from build123d import *

# Parameters (mm, degrees)
SKETCH1_R           = 11.2
SKETCH1_R_2         = 13
SKETCH1_R_3         = 1.45
SKETCH1_R_4         = 2.2
BOSS_EXTRUDE1_DEPTH = 5
BOSS_EXTRUDE2_DEPTH = 33
SKETCH1_4_R         = 13
SKETCH1_4_R_2       = 9.6
SKETCH1_4_R_3       = 8.6
SKETCH1_4_R_4       = 6
BOSS_EXTRUDE3_DEPTH = 3
SKETCH1_5_R         = 13
SKETCH1_5_R_2       = 9.6
SKETCH1_5_R_3       = 8.6
BOSS_EXTRUDE4_DEPTH = 8
SKETCH1_6_R         = 13
SKETCH1_6_R_2       = 9.6
BOSS_EXTRUDE5_DEPTH = 10
SKETCH2_R           = 2.2
CUT_EXTRUDE1_DEPTH  = 10
CHAMFER1_SIZE       = 4
CHAMFER2_SIZE       = 5


with BuildPart() as part:
    # Sketch1 → Boss-Extrude1 (new body)
    # profile 1 of 2: a face of its own
    with BuildSketch(Plane(origin=(0, 0, 0), x_dir=(1, 0, 0), z_dir=(0, 1, 0))):
        Polygon((-45, -45), (-45, -24), (-45, -21.4), (-71.4, -21.4), (-71.4, 21.4), (-45, 21.4), (-45, 24), (-45, 45), (45, 45), (45, 21), (76, 21), (76, -21), (45, -21), (45, -45), align=None)
        with Locations(Location((55, 0, 0), (0, 0, 270))):
            Circle(SKETCH1_R, mode=Mode.SUBTRACT)
        with Locations(Location((0, 0, 0), (0, 0, 270))):
            Circle(SKETCH1_R_2, mode=Mode.SUBTRACT)
        with Locations(Location((39.5, -15.5, 0), (0, 0, 270))):
            Circle(SKETCH1_R_3, mode=Mode.SUBTRACT)
        with Locations(Location((-35, -35, 0), (0, 0, 270))):
            Circle(SKETCH1_R_4, mode=Mode.SUBTRACT)
        with Locations(Location((-35, 35, 0), (0, 0, 270))):
            Circle(SKETCH1_R_4, mode=Mode.SUBTRACT)
        with Locations(Location((35, 35, 0), (0, 0, 270))):
            Circle(SKETCH1_R_4, mode=Mode.SUBTRACT)
        with Locations(Location((39.5, 15.5, 0), (0, 0, 270))):
            Circle(SKETCH1_R_3, mode=Mode.SUBTRACT)
        with Locations(Location((70.5, 15.5, 0), (0, 0, 270))):
            Circle(SKETCH1_R_3, mode=Mode.SUBTRACT)
        with Locations(Location((35, -35, 0), (0, 0, 270))):
            Circle(SKETCH1_R_4, mode=Mode.SUBTRACT)
        with Locations(Location((70.5, -15.5, 0), (0, 0, 270))):
            Circle(SKETCH1_R_3, mode=Mode.SUBTRACT)
    # profile 2 of 2: a face of its own
    with BuildSketch(Plane(origin=(0, 0, 0), x_dir=(1, 0, 0), z_dir=(0, 1, 0))):
        Polygon((-45, -24), (-74, -24), (-74, 24), (-45, 24), (-45, 21.4), (-71.4, 21.4), (-71.4, -21.4), (-45, -21.4), align=None)
    extrude(amount=BOSS_EXTRUDE1_DEPTH)

    # Sketch1_3 → Boss-Extrude2 (add)
    with BuildSketch(Plane(origin=(0, 0, 0), x_dir=(1, 0, 0), z_dir=(0, 1, 0))):
        Polygon((-45, -24), (-74, -24), (-74, 24), (-45, 24), (-45, 21.4), (-71.4, 21.4), (-71.4, -21.4), (-45, -21.4), align=None)
    extrude(amount=BOSS_EXTRUDE2_DEPTH)

    # Sketch1_4 → Boss-Extrude3 (add)
    # profile 1 of 3: a face of its own
    with BuildSketch(Plane(origin=(0, 0, 0), x_dir=(1, 0, 0), z_dir=(0, 1, 0))):
        with Locations(Location((0, 0, 0), (0, 0, 270))):
            Circle(SKETCH1_4_R)
        Circle(SKETCH1_4_R_2, mode=Mode.SUBTRACT)
    # profile 2 of 3: a face of its own
    with BuildSketch(Plane(origin=(0, 0, 0), x_dir=(1, 0, 0), z_dir=(0, 1, 0))):
        Circle(SKETCH1_4_R_2)
        Circle(SKETCH1_4_R_3, mode=Mode.SUBTRACT)
    # profile 3 of 3: a face of its own
    with BuildSketch(Plane(origin=(0, 0, 0), x_dir=(1, 0, 0), z_dir=(0, 1, 0))):
        Circle(SKETCH1_4_R_3)
        with Locations(Location((0, 0, 0), (0, 0, 270))):
            Circle(SKETCH1_4_R_4, mode=Mode.SUBTRACT)
    extrude(amount=BOSS_EXTRUDE3_DEPTH)

    # Sketch1_5 → Boss-Extrude4 (add)
    # profile 1 of 2: a face of its own
    with BuildSketch(Plane(origin=(0, 0, 0), x_dir=(1, 0, 0), z_dir=(0, 1, 0))):
        with Locations(Location((0, 0, 0), (0, 0, 270))):
            Circle(SKETCH1_5_R)
        Circle(SKETCH1_5_R_2, mode=Mode.SUBTRACT)
    # profile 2 of 2: a face of its own
    with BuildSketch(Plane(origin=(0, 0, 0), x_dir=(1, 0, 0), z_dir=(0, 1, 0))):
        Circle(SKETCH1_5_R_2)
        with Locations(Location((0, 0, 0), (0, 0, 270))):
            Circle(SKETCH1_5_R_3, mode=Mode.SUBTRACT)
    extrude(amount=BOSS_EXTRUDE4_DEPTH)

    # Sketch1_6 → Boss-Extrude5 (add)
    with BuildSketch(Plane(origin=(0, 0, 0), x_dir=(1, 0, 0), z_dir=(0, 1, 0))):
        with Locations(Location((0, 0, 0), (0, 0, 270))):
            Circle(SKETCH1_6_R)
        with Locations(Location((0, 0, 0), (0, 0, 270))):
            Circle(SKETCH1_6_R_2, mode=Mode.SUBTRACT)
    extrude(amount=BOSS_EXTRUDE5_DEPTH)

    # Sketch2 → Cut-Extrude1 (cut)
    with BuildSketch(Plane(origin=(-71.4, 0, 0), x_dir=(0, 0, -1), z_dir=(1, 0, 0))):
        with Locations((0, 19)):
            Circle(SKETCH2_R)
    extrude(amount=-CUT_EXTRUDE1_DEPTH, mode=Mode.SUBTRACT)

    # Chamfer1
    chamfer1_edges = [part.edges().sort_by_distance(p)[0] for p in [
        (-45, 2.5, -45),
        (45, 2.5, -45),
        (45, 2.5, -21),
        (76, 2.5, -21),
        (76, 2.5, 21),
        (45, 2.5, 21),
        (45, 2.5, 45),
        (-45, 2.5, 45),
    ]]
    chamfer(chamfer1_edges, length=CHAMFER1_SIZE)

    # Chamfer2
    chamfer2_edges = [part.edges().sort_by_distance(p)[0] for p in [
        (-45, 33, -22.7),
        (-45, 33, 22.7),
    ]]
    chamfer(chamfer2_edges, length=CHAMFER2_SIZE)


solid = part.part
CAD build for the part. Positions are in the model's coordinates, mm. A direction names the side the tool comes from. Coordinates: 2 decimals unless noted, no trailing zeros. Write each loop counter-clockwise with the first axis right and the second up, starting at its lowest first coordinate (ties: lowest second). Pieces come first, ordered by that corner, then holes. Notation, with made-up numbers: M 64.25,-39 L 117.25,-39 A18 cw 117.25,-11 Z; hole C -3,-11.75 d9. An arc over 180 degrees is marked long. Return JSON: item names as keys, results as strings.
Item 1: Two-plate mould, pull along X, no slides. Class faces 1 (the flat face through (-59, 16, 24)), 2 (the cylindrical face through (-37.148, 2.465, -35.477)), 3 (the flat face through (-74, 16, 0)), 4 (the flat face through (-71.4, 22, 0)): +X half, -X half, draft (parallel to the pull), parting line (faces both ways), or undercut.
Findings below:
{"face 1": "draft", "face 2": "undercut", "face 3": "-X half", "face 4": "undercut"}
Item 2: Probe line 1 (X direction, y = 8.85, z = 0); line 2 (X direction, y = 4.65, z = 0); line 3 (Z direction, x = 0.5, y = 4). List the from-to ranges inside material, lowest first. Write a range as from..to.
Findings below:
{"line 1": "x = -74..-71.4, -13..-9.6, 9.6..13", "line 2": "x = -74..-8.6, 8.6..43.8, 66.2..76", "line 3": "z = -45..-8.59, 8.59..45"}
Item 3: Slice it at D-D, the plane x = -54. Write the cut outline in (y, z), and give its area (3 significant figures).
Findings below:
{"outline": "M 0,-24 L 33,-24 L 33,-21.4 L 5,-21.4 L 5,21.4 L 33,21.4 L 33,24 L 0,24 Z", "area": "386 mm2"}
Item 4: Slice it at B-B, the plane x = 35. Write the cut outline in (y, z), and give its area (3 significant figures).
Findings below:
{"outline": "M 0,-45 L 5,-45 L 5,-37.2 L 0,-37.2 Z; M 0,-32.8 L 5,-32.8 L 5,32.8 L 0,32.8 Z; M 0,37.2 L 5,37.2 L 5,45 L 0,45 Z", "area": "406 mm2"}
Item 5: Slice it at A-A, the plane z = -15.5. Write the cut outline in (x, y).
Findings below:
{"outline": "M -74,0 L 38.05,0 L 38.05,5 L -71.4,5 L -71.4,33 L -74,33 Z; M 40.95,0 L 69.05,0 L 69.05,5 L 40.95,5 Z; M 71.95,0 L 76,0 L 76,5 L 71.95,5 Z"}
Item 6: Slice it at C-C, the plane y = 19. Write the cut outline in (x, z).
Findings below:
{"outline": "M -74,-24 L -45,-24 L -45,-21.4 L -71.4,-21.4 L -71.4,-2.2 L -74,-2.2 Z; M -74,2.2 L -71.4,2.2 L -71.4,21.4 L -45,21.4 L -45,24 L -74,24 Z"}
Item 7: Drop flat-ended pins along their axis: pin 1 Ø5.5 at (y, z) = (2, -30.5) entering from -X; pin 2 Ø5.5 at (y, z) = (3, 35.5) entering from +X; pin 3 Ø6 at (x, z) = (-4.5, 7.5) entering from +Y. Give the stop position or say it passes through.
Findings below:
{"pin 1": "stops at x = -45", "pin 2": "stops at x = 45", "pin 3": "stops at y = 10"}
Item 8: Which spindle directions (+Z, -Z, +X, -X, +Y, -Y) get a long thin tool onto all of the face, cutting with end or side? Do faces 5 (the cylindrical face through (-7.91, 7.465, -10.316)), 6 (the flat face through (-10, 10, -1)), 7 (the flat face through (74, 2, 19)), 8 (the flat face through (45, 2, -33)). Say none if no direction does.
Findings below:
{"face 5": "+Y", "face 6": "+Z, -Z, +X, +Y", "face 7": "+Z, +X, +Y, -Y", "face 8": "-Z, +X, +Y, -Y"}
